```python
from build123d import *

# Parameters (mm, degrees)
SKETCH_1_R      = 15
EXTRUDE_1_DEPTH = 19.5
SKETCH_2_R      = 10
EXTRUDE_2_DEPTH = 1
SKETCH_3_R      = 7.5
EXTRUDE_3_DEPTH = 11
M3X0_52_D       = 2.5
M3X0_51_D       = 2.5
M3X0_51_DEPTH   = 8
M3X0_51_TIP     = 0.751075774


with BuildPart() as part:
    # Эскиз1 → Бобышка-Вытянуть1 (new body)
    with BuildSketch(Plane.XY):
        Circle(SKETCH_1_R)
    extrude(amount=EXTRUDE_1_DEPTH)

    # Эскиз2 → Бобышка-Вытянуть2 (add)
    with BuildSketch(Plane.XY.offset(19.5)):
        Circle(SKETCH_2_R)
    extrude(amount=EXTRUDE_2_DEPTH)

    # Эскиз3 → Бобышка-Вытянуть3 (add)
    with BuildSketch(Plane.XY.offset(20.5)):
        Circle(SKETCH_3_R)
    extrude(amount=EXTRUDE_3_DEPTH)

    # Отверстие обработанное метчиком M3x0.52 (through all)
    with Locations(Plane(origin=(0, 0, 0), x_dir=(-1, 0, 0), z_dir=(0, 0, -1))):
        with Locations((0, 10), (10, 0), (-10, 0), (0, -10)):
            Hole(M3X0_52_D / 2)

    # Отверстие обработанное метчиком M3x0.51
    with Locations(Plane.XY.offset(31.5)):
        with Locations((-2.828427125, -2.828427125), (2.828427125, 2.828427125)):
            Hole(M3X0_51_D / 2, depth=M3X0_51_DEPTH)
            with Locations((0, 0, -(M3X0_51_DEPTH + M3X0_51_TIP / 2))):  # 118° drill point
                Cone(0, M3X0_51_D / 2, M3X0_51_TIP, mode=Mode.SUBTRACT)


solid = part.part
```
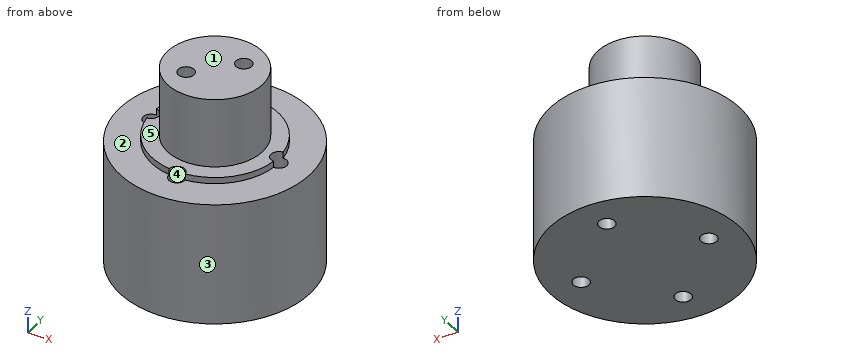
The model under review builds one solid part; all positions refer to its coordinate system, in mm. Face numbers are marked on the shaded views. A direction names the side the tool comes from. Give positions to 0.01 mm unless a question says otherwise; leave off trailing zeros. Write each loop counter-clockwise with the first axis right and the second up, starting at its lowest first coordinate (ties: lowest second). Pieces come first, ordered by that corner, then holes. Notation, with made-up numbers: (52, -2.5) - (99, -2.5) arc R20 ccw to (99, 8.5) - close; hole circle Ø8 at (17, 85). An arc over 180 degrees is marked (long way). Answer in a Markdown table with one row per item. Add a question column.
1. Draft analysis for pull direction Y (two halves, no side actions). For the marked faces 3, 4 and 5, state which applies: +Y half, -Y half, draft (parallel to the pull), parting line (faces both ways), or undercut.
2. Tool access review of the marked faces 1 and 2: name each direction out of +Z, -Z, +X, -X, +Y, -Y from which nothing blocks a thin tool from reaching the whole face with its end or side.
3. We need section D-D on y = -4.75. Write out the cut boundary in (x, z).
4. We need section A-A on y = 0. Write out the cut boundary in (x, z).
5. We need section C-C on x = 6.5. Write out the cut boundary in (y, z), then the cut area to 3 significant figures.
6. Wall thickness on line 1 along Y through (x, z) = (0, 12.5); line 2 along X through (y, z) = (-1, 4); line 3 along Z through (x, y) = (5.5, -13): over which ranges is each line inside the solid? List them lowest first. Write a range as [from, to].
7. Insertion check: P1, Ø2, axis at x = -4.5, z = 24, coming from the -Y side; P2, Ø10, axis at x = 10, z = 28, coming from the +Y side; P3, Ø4, axis at x = 0, y = -10, coming from the +Z side; P4, Ø1.5, axis at x = -10, y = 0, coming from the -Z side. Each pin has a flat end and moves straight along its axis. Give the tip position at first contact, or say it passes through.
8. We need section B-B on z = 6.5. Write out the cut boundary in (x, y), then the cut area to 3 significant figures.
Ans:
| question | item | result |
|---|---|---|
| 1 | face 3 | parting line |
| 1 | face 4 | undercut |
| 1 | face 5 | draft |
| 2 | face 1 | +Z, +X, -X, +Y, -Y |
| 2 | face 2 | +Z |
| 3 | outline | (-14.23, 0) - (14.23, 0) - (14.23, 19.5) - (8.8, 19.5) - (8.8, 20.5) - (5.8, 20.5) - (5.8, 31.5) - (-5.8, 31.5) - (-5.8, 20.5) - (-8.8, 20.5) - (-8.8, 19.5) - (-14.23, 19.5) - close |
| 4 | outline | (-15, 0) - (-11.25, 0) - (-11.25, 19.5) - (-15, 19.5) - close; (-8.75, 0) - (8.75, 0) - (8.75, 20.5) - (7.5, 20.5) - (7.5, 31.5) - (-7.5, 31.5) - (-7.5, 20.5) - (-8.75, 20.5) - close; (11.25, 0) - (15, 0) - (15, 19.5) - (11.25, 19.5) - close |
| 5 | outline | (-13.52, 0) - (13.52, 0) - (13.52, 19.5) - (7.6, 19.5) - (7.6, 20.5) - (3.74, 20.5) - (3.74, 31.5) - (-3.74, 31.5) - (-3.74, 20.5) - (-7.6, 20.5) - (-7.6, 19.5) - (-13.52, 19.5) - close |
| 5 | area | 625 mm^2 |
| 6 | line 1 | y = [-15, -11.25], [-8.75, 8.75], [11.25, 15] |
| 6 | line 2 | x = [-14.97, -10.75], [-9.25, 9.25], [10.75, 14.97] |
| 6 | line 3 | z = [0, 19.5] |
| 7 | P1 | stops at y = -6.63 |
| 7 | P2 | stops at y = 5.59 |
| 7 | P3 | stops at z = 20.5 |
| 7 | P4 | passes through |
| 8 | outline | circle Ø30 at (0, 0); hole circle Ø2.5 at (-10, 0); hole circle Ø2.5 at (0, -10); hole circle Ø2.5 at (0, 10); hole circle Ø2.5 at (10, 0) |
| 8 | area | 687 mm^2 |
